```python
from build123d import *

# Parameters (mm, degrees)
SKETCH1_W           = 100
SKETCH1_H           = 100
BOSS_EXTRUDE1_DEPTH = 53.5
SKETCH2_R           = 2.5
SKETCH2_W           = 12.6
SKETCH2_H           = 3.072407599
BOSS_EXTRUDE2_DEPTH = 4
CUT_EXTRUDE1_DEPTH  = 47.5
FILLET1_R           = 3.25
FILLET2_R           = 3
SKETCH4_R           = 1.625
CUT_EXTRUDE2_DEPTH  = 14
FILLET3_R           = 3


with BuildPart() as part:
    # Sketch1 → Boss-Extrude1 (new body)
    with BuildSketch(Plane(origin=(0, 0, 0), x_dir=(1, 0, 0), z_dir=(0, 1, 0))):
        Rectangle(SKETCH1_W, SKETCH1_H)
    extrude(amount=BOSS_EXTRUDE1_DEPTH)

    # Sketch2 → Boss-Extrude2 (add)
    # profile 1 of 8: a face of its own
    with BuildSketch(Plane.XZ):
        with BuildLine():
            Line((33.15, -50), (20.55, -50))
            Line((20.55, -50), (20.55, -56.973787721))
            ThreePointArc((20.55, -56.973787721), (26.85, -63.273787721), (33.15, -56.973787721))
            Line((33.15, -56.973787721), (33.15, -50))
        make_face()
        with Locations(Location((26.85, -56.973787721, 0), (0, 0, 270))):
            Circle(SKETCH2_R, mode=Mode.SUBTRACT)
    # profile 2 of 8: a face of its own
    with BuildSketch(Plane.XZ):
        with BuildLine():
            Line((-20.55, -56.973787721), (-20.55, -50))
            Line((-20.55, -50), (-33.15, -50))
            Line((-33.15, -50), (-33.15, -56.973787721))
            ThreePointArc((-33.15, -56.973787721), (-26.85, -63.273787721), (-20.55, -56.973787721))
        make_face()
        with Locations(Location((-26.85, -56.973787721, 0), (0, 0, 270))):
            Circle(SKETCH2_R, mode=Mode.SUBTRACT)
    # profile 3 of 8: a face of its own
    with BuildSketch(Plane.XZ):
        with Locations((-26.85, 48.4637962)):
            Rectangle(SKETCH2_W, SKETCH2_H)
    # profile 4 of 8: a face of its own
    with BuildSketch(Plane.XZ):
        with BuildLine():
            Line((-33.15, 50), (-20.55, 50))
            Line((-20.55, 50), (-20.55, 56.973787721))
            ThreePointArc((-20.55, 56.973787721), (-26.85, 63.273787721), (-33.15, 56.973787721))
            Line((-33.15, 56.973787721), (-33.15, 50))
        make_face()
        with Locations(Location((-26.85, 56.973787721, 0), (0, 0, 270))):
            Circle(SKETCH2_R, mode=Mode.SUBTRACT)
    # profile 5 of 8: a face of its own
    with BuildSketch(Plane.XZ):
        with BuildLine():
            Line((20.55, 56.973787721), (20.55, 50))
            Line((20.55, 50), (33.15, 50))
            Line((33.15, 50), (33.15, 56.973787721))
            ThreePointArc((33.15, 56.973787721), (26.85, 63.273787721), (20.55, 56.973787721))
        make_face()
        with Locations(Location((26.85, 56.973787721, 0), (0, 0, 270))):
            Circle(SKETCH2_R, mode=Mode.SUBTRACT)
    # profile 6 of 8: a face of its own
    with BuildSketch(Plane.XZ):
        with Locations((26.85, 48.4637962)):
            Rectangle(SKETCH2_W, SKETCH2_H)
    # profile 7 of 8: a face of its own
    with BuildSketch(Plane.XZ):
        with Locations((26.85, -48.4637962)):
            Rectangle(SKETCH2_W, SKETCH2_H)
    # profile 8 of 8: a face of its own
    with BuildSketch(Plane.XZ):
        with Locations((-26.85, -48.4637962)):
            Rectangle(SKETCH2_W, SKETCH2_H)
    extrude(amount=-BOSS_EXTRUDE2_DEPTH)

    # Sketch3 → Cut-Extrude1 (cut)
    with BuildSketch(Plane(origin=(0, 53.5, 0), x_dir=(1, 0, 0), z_dir=(0, 1, 0))):
        Polygon((35.565, 48), (-35.565, 48), (-48, 35.565), (-48, -35.565), (-35.565, -48), (35.565, -48), (48, -35.565), (48, 35.565), align=None)
    extrude(amount=-CUT_EXTRUDE1_DEPTH, mode=Mode.SUBTRACT)

    # Fillet1
    fillet1_edges = [part.edges().sort_by_distance(p)[0] for p in [
        (50, 26.75, 50),
        (-50, 26.75, 50),
        (-50, 26.75, -50),
        (50, 26.75, -50),
    ]]
    fillet(fillet1_edges, radius=FILLET1_R)

    # Fillet2
    fillet2_edges = [part.edges().sort_by_distance(p)[0] for p in [
        (-26.85, 4, 50),
        (26.85, 4, 50),
        (26.85, 4, -50),
        (-26.85, 4, -50),
    ]]
    fillet(fillet2_edges, radius=FILLET2_R)

    # Sketch4 → Cut-Extrude2 (cut)
    with BuildSketch(Plane(origin=(0, 53.5, 0), x_dir=(1, 0, 0), z_dir=(0, 1, 0))):
        with Locations(Location((-46.75, 46.75, 0), (0, 0, 270))):
            Circle(SKETCH4_R)
        with Locations(Location((46.75, 46.75, 0), (0, 0, 270))):
            Circle(SKETCH4_R)
        with Locations(Location((46.75, -46.75, 0), (0, 0, 270))):
            Circle(SKETCH4_R)
        with Locations(Location((-46.75, -46.75, 0), (0, 0, 270))):
            Circle(SKETCH4_R)
    extrude(amount=-CUT_EXTRUDE2_DEPTH, mode=Mode.SUBTRACT)

    # Fillet3
    fillet3_edges = [part.edges().sort_by_distance(p)[0] for p in [
        (50, 0, 0),
        (39.95, 0, -50),
        (-39.95, 0, 50),
        (-50, 0, 0),
        (49.048097039, 0, -49.048097039),
        (-49.048097039, 0, -49.048097039),
        (-49.048097039, 0, 49.048097039),
        (49.048097039, 0, 49.048097039),
        (0, 0, 50),
        (39.95, 0, 50),
        (0, 0, -50),
        (-39.95, 0, -50),
    ]]
    fillet(fillet3_edges, radius=FILLET3_R)


solid = part.part
```
Can you work these out from the model? Positions are in its coordinate system, mm. A direction names the side the tool comes from. Coordinates: 2 decimals unless noted, no trailing zeros. Loops run counter-clockwise (first coordinate to the right, second up) from the corner with the lowest first, then second, coordinate; pieces in that order, holes last.
1) Imagine slicing it at C-C on x = -26.85. List the corners of the cut face in (y, z) for me, plus the area to 3 significant figures.
2) Imagine slicing it at A-A on y = 16. List the corners of the cut face in (x, z) for me (3 decimals).
3) Imagine slicing it at D-D on z = -25.5. List the corners of the cut face in (x, y) for me.
4) I need wall thicknesses on probe 1 along X at (y, z) = (35.5, 34.5); probe 2 along Z at (x, y) = (-26, 1). Which ranges of each line are inside material? Lowest first, please.
5) Imagine slicing it at B-B on x = -16. List the corners of the cut face in (y, z) for me.
6) For pin 1 (12 mm diameter, centred on x = -12.5, z = 10.5, fed in from +Y); pin 2 (4.5 mm diameter, centred on x = 26.85, z = 56.97, fed in from -Y); pin 3 (2 mm diameter, centred on y = 3, z = -50, fed in from -X); pin 4 (3 mm diameter, centred on x = 22.5, y = 11, fed in from +Z), each with a flat end and sliding along its axis, tell me the tip position at first contact or that it passes through.
7) Thinking about a two-plate mould opening in Z: for faces 4 (the flat face through (-20.55, 2, -53)), 5 (the cylindrical face through (-39.85, 0.86, 49.1)), 6 (the cylindrical face through (39.85, 0.86, -49.1)), 7 (the flat face through (-47, 39.5, -47)), which applies, pulls with the +Z half, pulls with the -Z half, needs draft (parallel to the pull), parting line crosses it, or undercut?
8) Which directions (+Z, -Z, +X, -X, +Y, -Y) give clear straight access to the entire face, cutting with the end or side of a thin tool? Please do faces 1 (the flat face through (25, 4, -59)), 2 (the cylindrical face through (-49.1, 0.86, 0.65)), 3 (the flat face through (-48, 30, 0)).
Completed:
1. outline: (0, -63.27) - (4, -63.27) - (4, -59.47) - (0, -59.47) - close; (0, -54.47) - (4, -54.47) - (4, -53) arc R3 cw to (7, -50) - (53.5, -50) - (53.5, -48) - (6, -48) - (6, 48) - (53.5, 48) - (53.5, 50) - (7, 50) arc R3 cw to (4, 53) - (4, 54.47) - (0, 54.47) - close; (0, 59.47) - (4, 59.47) - (4, 63.27) - (0, 63.27) - close
1. area: 860 mm2
2. outline: (-50, -46.75) arc R3.25 ccw to (-46.75, -50) - (46.75, -50) arc R3.25 ccw to (50, -46.75) - (50, 46.75) arc R3.25 ccw to (46.75, 50) - (-46.75, 50) arc R3.25 ccw to (-50, 46.75) - close; hole (-48, -35.565) - (-35.565, -48) - (35.565, -48) - (48, -35.565) - (48, 35.565) - (35.565, 48) - (-35.565, 48) - (-48, 35.565) - close
3. outline: (-50, 3) arc R3 ccw to (-47, 0) - (47, 0) arc R3 ccw to (50, 3) - (50, 53.5) - (48, 53.5) - (48, 6) - (-48, 6) - (-48, 53.5) - (-50, 53.5) - close
4. probe 1: x = -50 to -48, 48 to 50
4. probe 2: z = -63.22 to -59.32, -54.62 to 54.62, 59.32 to 63.22
5. outline: (0, -47) arc R3 ccw to (3, -50) - (53.5, -50) - (53.5, -48) - (6, -48) - (6, 48) - (53.5, 48) - (53.5, 50) - (3, 50) arc R3 ccw to (0, 47) - close
6. pin 1: stops at y = 6
6. pin 2: passes through
6. pin 3: stops at x = -49.1
6. pin 4: stops at z = 50
7. face 4: needs draft
7. face 5: pulls with the +Z half
7. face 6: pulls with the -Z half
7. face 7: undercut
8. face 1: -Z, +X, -X, +Y
8. face 2: +Z, -Z, -X, -Y
8. face 3: +Y
